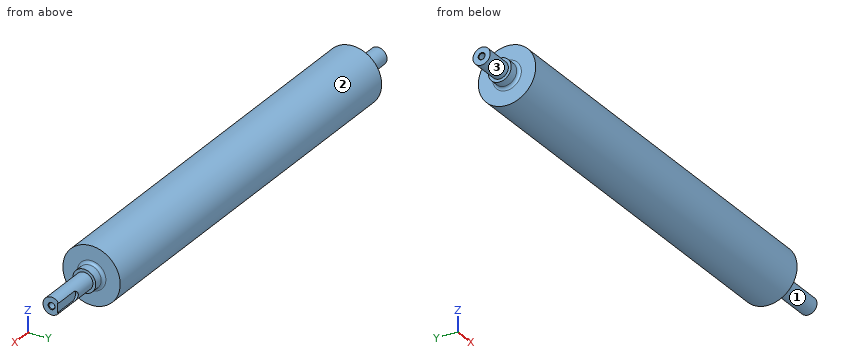
from build123d import *

# Parameters (mm, degrees)
FILLET1_R                              = 5
M12_TAPPED_HOLE1_D                     = 10.2
M12_TAPPED_HOLE1_DEPTH                 = 29.25
M12_TAPPED_HOLE1_CSINK_D               = 12.05
M12_TAPPED_HOLE1_CSINK_ANGLE           = 90
M12_TAPPED_HOLE1_TIP                   = 3.064389157
M12_TAPPED_HOLE1_ON_FACE_2_D           = 10.2
M12_TAPPED_HOLE1_ON_FACE_2_DEPTH       = 29.25
M12_TAPPED_HOLE1_ON_FACE_2_CSINK_D     = 12.05
M12_TAPPED_HOLE1_ON_FACE_2_CSINK_ANGLE = 90
M12_TAPPED_HOLE1_ON_FACE_2_TIP         = 3.064389157
CUT_EXTRUDE1_DEPTH                     = 5


with BuildPart() as part:
    # Sketch1 → Revolve1 (revolve)
    with BuildSketch(Plane.XY):
        Polygon((0, 0), (0, 15), (50, 15), (50, 20), (70, 20), (70, 50), (790, 50), (790, 20), (810, 20), (810, 15), (900, 15), (900, 0), align=None)
    revolve(axis=Axis((900, 0, 0), (-1, 0, 0)))

    # Fillet1
    fillet1_edges = [part.edges().sort_by_distance(p)[0] for p in [
        (790, -20, 0),
        (70, -20, 0),
    ]]
    fillet(fillet1_edges, radius=FILLET1_R)

    # M12 Tapped Hole1
    with Locations(Plane.YZ.offset(900)):
        with Locations((0, 0)):
            CounterSinkHole(M12_TAPPED_HOLE1_D / 2, M12_TAPPED_HOLE1_CSINK_D / 2, depth=M12_TAPPED_HOLE1_DEPTH, counter_sink_angle=M12_TAPPED_HOLE1_CSINK_ANGLE)
            with Locations((0, 0, -(M12_TAPPED_HOLE1_DEPTH + M12_TAPPED_HOLE1_TIP / 2))):  # 118° drill point
                Cone(0, M12_TAPPED_HOLE1_D / 2, M12_TAPPED_HOLE1_TIP, mode=Mode.SUBTRACT)

    # M12 Tapped Hole1 on face 2
    with Locations(Plane(origin=(0, 0, 0), x_dir=(0, 0, -1), z_dir=(-1, 0, 0))):
        with Locations((0, 0)):
            CounterSinkHole(M12_TAPPED_HOLE1_ON_FACE_2_D / 2, M12_TAPPED_HOLE1_ON_FACE_2_CSINK_D / 2, depth=M12_TAPPED_HOLE1_ON_FACE_2_DEPTH, counter_sink_angle=M12_TAPPED_HOLE1_ON_FACE_2_CSINK_ANGLE)
            with Locations((0, 0, -(M12_TAPPED_HOLE1_ON_FACE_2_DEPTH + M12_TAPPED_HOLE1_ON_FACE_2_TIP / 2))):  # 118° drill point
                Cone(0, M12_TAPPED_HOLE1_ON_FACE_2_D / 2, M12_TAPPED_HOLE1_ON_FACE_2_TIP, mode=Mode.SUBTRACT)

    # Sketch3 → Cut-Extrude1 (cut)
    with BuildSketch(Plane(origin=(0, 15, 0), x_dir=(1, 0, 0), z_dir=(0, 1, 0))):
        with BuildLine():
            Line((858.516691337, 8.516691337), (900, 8.516691337))
            ThreePointArc((900, 8.516691337), (908.516691337, 0), (900, -8.516691337))
            Line((900, -8.516691337), (858.516691337, -8.516691337))
            ThreePointArc((858.516691337, -8.516691337), (850, 0), (858.516691337, 8.516691337))
        make_face()
    extrude(amount=-CUT_EXTRUDE1_DEPTH, mode=Mode.SUBTRACT)


solid = part.part
The listing builds one solid part. Answer for the finished solid, in the listing's coordinates (mm). Face numbers are marked on the shaded views. A direction names the side the tool comes from. Coordinates: 2 decimals unless noted, no trailing zeros. Loops run counter-clockwise (first coordinate to the right, second up) from the corner with the lowest first, then second, coordinate; pieces in that order, holes last. Notation, with made-up numbers: M -37.5,-31.75 L -32.5,-31.75 A26 cw -32.5,4.25 Z; hole C -35,0 d11. An arc over 180 degrees is marked long. Answer in a Markdown table with one row per item.
1) Find section B-B (z = -42.5). Determine the outline of the cut face in (x, y), then the cut area to 3 significant figures.
Answers below:
| item | result |
|---|---|
| outline | M 70,-26.34 L 790,-26.34 L 790,26.34 L 70,26.34 Z |
| area | 37,900 mm^2 |
2) Find section C-C (y = -37.5). Determine the outline of the cut face in (x, z), then the cut area to 3 significant figures.
Answers below:
| item | result |
|---|---|
| outline | M 70,-33.07 L 790,-33.07 L 790,33.07 L 70,33.07 Z |
| area | 47,600 mm^2 |
3) Given pin 1 (6 mm diameter, centred on y = 0, z = 0, fed in from -X); pin 2 (1.5 mm diameter, centred on x = 361.5, z = -13, fed in from +Y); pin 3 (4 mm diameter, centred on x = 387.5, z = 18.5, fed in from +Y), each flat-ended and moving along its own axis, determine where each tip first touches the part or whether it passes through.
Answers below:
| item | result |
|---|---|
| pin 1 | x = 30.51 |
| pin 2 | y = 48.48 |
| pin 3 | y = 47.2 |
4) Find the intervals of material crossed by probe 1 along Y at (x, z) = (893.25, 0); probe 2 along Y at (x, z) = (11, 0), in increasing order.
Answers below:
| item | result |
|---|---|
| probe 1 | -15 to -5.1, 5.1 to 10 |
| probe 2 | -15 to -5.1, 5.1 to 15 |
5) Find section A-A (x = 519). Determine the outline of the cut face in (y, z).
Answers below:
| item | result |
|---|---|
| outline | C 0,0 d100 |
6) Which of the six approach directions +Z, -Z, +X, -X, +Y, -Y give full straight-line access (tool end or side, diameter ignored) to the marked faces 1, 2 and 3?
Answers below:
| item | result |
|---|---|
| face 1 | +X |
| face 2 | +X, -X |
| face 3 | -X |
